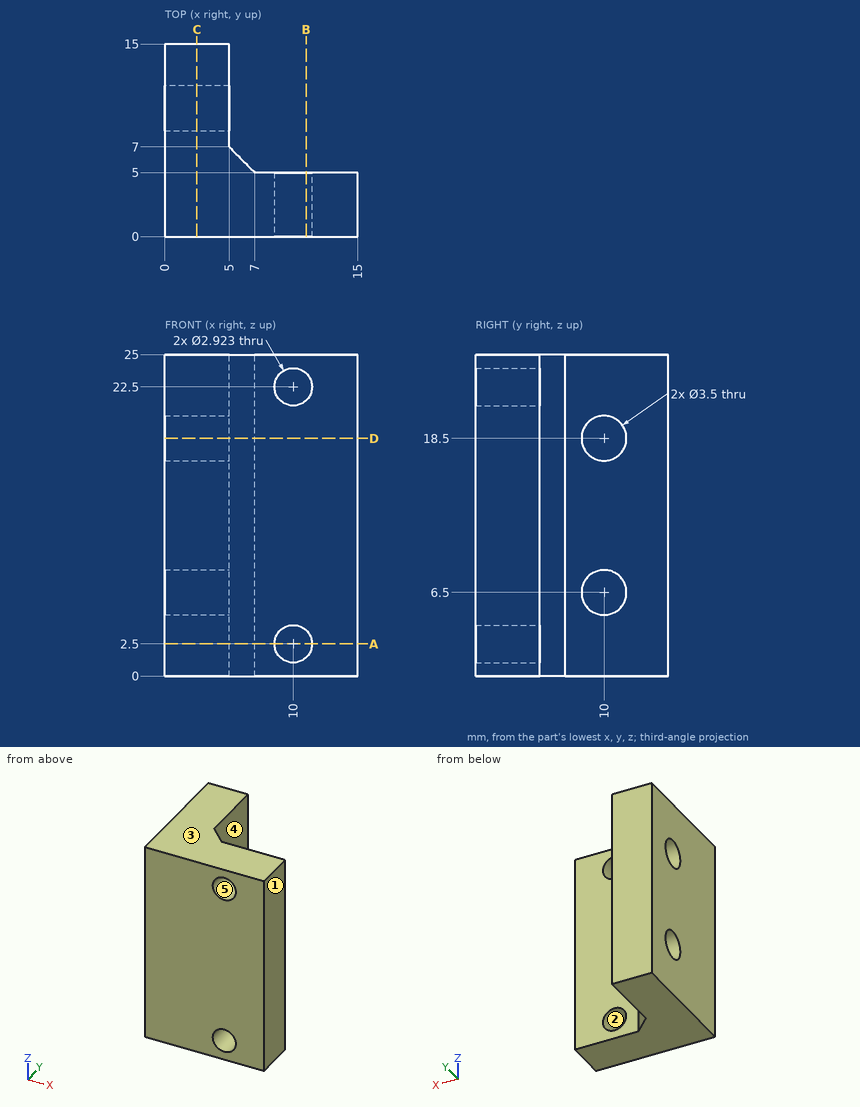
Check sheet for the drawn part. Datum: minimum x, y, z corner. Units: mm. A direction names the side the tool comes from. Round coordinates to 2 decimals unless told otherwise and drop trailing zeros. Loops run counter-clockwise (first coordinate to the right, second up) from the corner with the lowest first, then second, coordinate; pieces in that order, holes last.
Item 1: Cross-section at C-C on x = 2.5. Record the boundary of the cut face in (y, z), then the cut area to 3 significant figures.
Item 2: Cross-section at D-D on z = 18.5. Record the boundary of the cut face in (x, y).
Item 3: Gauge pin test, flat ends, axial feed: pin 1 (4 mm diameter, centred on y = 10, z = 6.5, fed in from +X); pin 2 (4 mm diameter, centred on x = 11.5, z = 16.5, fed in from +Y); pin 3 (3 mm diameter, centred on x = 7, z = 4, fed in from +Y). Record the tip position at first contact, or that the pin passes through.
Item 4: Cross-section at A-A on z = 2.5. Record the boundary of the cut face in (x, y).
Item 5: Mould release check, pull along Z, two halves, no side actions. Record for the marked faces 1, 2 and 3: pulls with the +Z half, pulls with the -Z half, needs draft (parallel to the pull), parting line crosses it, or undercut.
Item 6: Cross-section at B-B on x = 11. Record the boundary of the cut face in (y, z) (1 decimal), then the cut area to 3 significant figures.
Item 7: Access from +Z, -Z, +X, -X, +Y, -Y to the whole of each face (thin tool, end or side, straight path). Record for the marked faces 4 and 5.
Item 8: Thickness scan on line 1 (Z direction, x = 2.6, y = 10); line 2 (Z direction, x = 10, y = 3.75); line 3 (X direction, y = 12.5, z = 12.75). Record the ranges inside material, lowest first.
Answer sheet:
1. outline: (0, 0) - (15, 0) - (15, 25) - (0, 25) - close; hole circle Ø3.5 at (10, 6.5); hole circle Ø3.5 at (10, 18.5)
1. area: 356 mm2
2. outline: (0, 0) - (15, 0) - (15, 5) - (7, 5) - (5, 7) - (5, 8.25) - (0, 8.25) - close; (0, 11.75) - (5, 11.75) - (5, 15) - (0, 15) - close
3. pin 1: stops at x = 5
3. pin 2: stops at y = 5
3. pin 3: stops at y = 6.5
4. outline: (0, 0) - (8.54, 0) - (8.54, 5) - (7, 5) - (5, 7) - (5, 15) - (0, 15) - close; (11.46, 0) - (15, 0) - (15, 5) - (11.46, 5) - close
5. face 1: needs draft
5. face 2: undercut
5. face 3: pulls with the +Z half
6. outline: (0, 0) - (5, 0) - (5, 1.4) - (0, 1.4) - close; (0, 3.6) - (5, 3.6) - (5, 21.4) - (0, 21.4) - close; (0, 23.6) - (5, 23.6) - (5, 25) - (0, 25) - close
6. area: 104 mm2
7. face 4: +Z, -Z, +X, +Y
7. face 5: +Y, -Y
8. line 1: z = 0 to 4.75, 8.25 to 16.75, 20.25 to 25
8. line 2: z = 0 to 1.04, 3.96 to 21.04, 23.96 to 25
8. line 3: x = 0 to 5
